Geometry check sheet. Reference: the model listing, model coordinates, mm. A direction names the side the tool comes from. Coordinates: 2 decimals unless noted, no trailing zeros. Write each loop counter-clockwise with the first axis right and the second up, starting at its lowest first coordinate (ties: lowest second). Pieces come first, ordered by that corner, then holes. Notation, with made-up numbers: (74, -10.5) - (98, -10.5) arc R19 cw to (98, 24.5) - close; hole circle Ø2 at (-32, 67.25). An arc over 180 degrees is marked (long way). Answer as a JSON object with one key per item and string values. Group by question number.
from build123d import *

# Parameters (mm, degrees)
SKIZZE1_R                       = 50
AUFSATZ_LINEAR_AUSTRAGEN1_DEPTH = 3
AUFSATZ_LINEAR_AUSTRAGEN2_DEPTH = 28.85
SCHNITT_LINEAR_AUSTRAGEN1_DEPTH = 28.85


with BuildPart() as part:
    # Skizze1 → Aufsatz-Linear austragen1 (new body)
    with BuildSketch(Plane(origin=(0, 0, 0), x_dir=(1, 0, 0), z_dir=(0, 1, 0))):
        with Locations(Location((0, 0, 0), (0, 0, 270))):
            Circle(SKIZZE1_R)
    extrude(amount=AUFSATZ_LINEAR_AUSTRAGEN1_DEPTH)

    # Skizze2 → Aufsatz-Linear austragen2 (add)
    with BuildSketch(Plane(origin=(0, 3, 0), x_dir=(1, 0, 0), z_dir=(0, 1, 0))):
        Polygon((20.4, 4), (24.4, 4), (24.4, 11.2), (-24.4, 11.2), (-24.4, -11.2), (24.4, -11.2), (24.4, -4), (20.4, -4), (20.4, -10.2), (-20.4, -10.2), (-20.4, 10.2), (20.4, 10.2), align=None)
    extrude(amount=AUFSATZ_LINEAR_AUSTRAGEN2_DEPTH)

    # Skizze3 → Schnitt-Linear austragen1 (cut)
    with BuildSketch(Plane.XY.offset(11.2)):
        Polygon((-19.4, 31.85), (0, 7.681220191), (19.4, 31.85), align=None)
    extrude(amount=-SCHNITT_LINEAR_AUSTRAGEN1_DEPTH, mode=Mode.SUBTRACT)


solid = part.part
(1) Set-up check for faces 4 (the face through (-20.4, 17, 0)), 5 (the face through (6, 14, -11.2)), 6 (the face through (-9.836, 19.935, 10.707)): record each of +Z, -Z, +X, -X, +Y, -Y from which the full face is reachable in a straight line by a thin tool's end or side.
(2) Material ranges on L1, parallel to Z at x = -4, y = 12; L2, parallel to Z at x = 24, y = 5; L3, parallel to X at y = 28.5, z = -9.5, recorded low to high. Write a range as [from, to].
(3) Gauge pin test, flat ends, axial feed: pin 1 (6.5 mm diameter, centred on y = 18.5, z = -5, fed in from -X); pin 2 (8.5 mm diameter, centred on x = -0.5, y = 14.5, fed in from -Z); pin 3 (14.5 mm diameter, centred on x = -5, y = 17, fed in from +Z). Record the tip position at first contact, or that the pin passes through.
(4) Section check D-D (x = 8). Record the cut outline in (y, z).
(5) Section check C-C (x = -5). Record the cut outline in (y, z).
(6) Draft check along X on faces 1 (the face through (22, 17, 4)), 2 (the face through (24.4, 17, 8)), 3 (the face through (-9.836, 19.935, -10.693)). Enter one of: +X half, -X half, draft (parallel to the pull), parting line (faces both ways), or undercut.
(7) Section check B-B (z = 0). Record the cut outline in (x, y), and give its area (3 significant figures).
(8) Section check A-A (y = 22). Record the cut outline in (x, z).
Conclusion:
{
 "1": {"face 4": "+Y", "face 5": "-Z, +X, -X, +Y", "face 6": "+Z, -Z, +Y"},
 "2": {"L1": "z = [-11.2, -10.2], [10.2, 11.2]", "L2": "z = [-11.2, -4], [4, 11.2]", "L3": "x = [-24.4, -20.4], [20.4, 24.4]"},
 "3": {"pin 1": "stops at x = -24.4", "pin 2": "stops at z = -11.2", "pin 3": "stops at z = 11.2"},
 "4": {"outline": "(0, -49.36) - (3, -49.36) - (3, -11.2) - (17.65, -11.2) - (17.65, -10.2) - (3, -10.2) - (3, 10.2) - (17.65, 10.2) - (17.65, 11.2) - (3, 11.2) - (3, 49.36) - (0, 49.36) - close"},
 "5": {"outline": "(0, -49.75) - (3, -49.75) - (3, -11.2) - (13.91, -11.2) - (13.91, -10.2) - (3, -10.2) - (3, 10.2) - (13.91, 10.2) - (13.91, 11.2) - (3, 11.2) - (3, 49.75) - (0, 49.75) - close"},
 "6": {"face 1": "draft", "face 2": "+X half", "face 3": "undercut"},
 "7": {"outline": "(-50, 0) - (50, 0) - (50, 3) - (-20.4, 3) - (-20.4, 31.85) - (-24.4, 31.85) - (-24.4, 3) - (-50, 3) - close", "area": "415 mm^2"},
 "8": {"outline": "(-24.4, -11.2) - (-11.49, -11.2) - (-11.49, -10.2) - (-20.4, -10.2) - (-20.4, 10.2) - (-11.49, 10.2) - (-11.49, 11.2) - (-24.4, 11.2) - close; (11.49, -11.2) - (24.4, -11.2) - (24.4, -4) - (20.4, -4) - (20.4, -10.2) - (11.49, -10.2) - close; (11.49, 10.2) - (20.4, 10.2) - (20.4, 4) - (24.4, 4) - (24.4, 11.2) - (11.49, 11.2) - close"}
}
